Geometry: final body of the model. Coordinates: model frame, mm. A direction names the side the tool comes from. Give positions to 0.01 mm unless a question says otherwise; leave off trailing zeros. Write each loop counter-clockwise with the first axis right and the second up, starting at its lowest first coordinate (ties: lowest second). Pieces come first, ordered by that corner, then holes.
Q1. Cut plane C-C on y = 38. Return the cut outline in (x, z), plus the area to 3 significant figures.
Q2. Draft query along Z for faces 5 (the face through (99.254, 57.916, -4.251)), 6 (the face through (-38, 5, 16)), 7 (the face through (-39, 0, 0)), 8 (the face through (116, 41, -25)). Return one class per face: pulls with the +Z half, pulls with the -Z half, needs draft (parallel to the pull), parting line crosses it, or undercut.
Q3. Cut plane D-D on x = 120.5. Return the cut outline in (y, z).
Q4. Pin query (flat end, axial travel): pin 1 (11 mm diameter, centred on x = 91.5, y = 38.5, fed in from -Z); pin 2 (8 mm diameter, centred on y = 46, z = -12.5, fed in from -X); pin 3 (19 mm diameter, centred on x = 13.5, z = 35, fed in from -Y); pin 4 (18 mm diameter, centred on x = 89, z = 0, fed in from -Y). Return the tip coordinate at first contact, or that it passes through.
Q5. Line query: L1, parallel to Z at x = 0, y = 45; L2, parallel to Z at x = 89, y = 54; L3, parallel to Y at x = 21, z = -33.5. Output: solid intervals per line, ascending.
Q6. Cut plane A-A on x = 89. Return the cut outline in (y, z), plus the area to 3 significant figures.
Q7. Cut plane B-B on z = 0. Return the cut outline in (x, y), plus the area to 3 significant figures.
Q8. Reachability of faces 1 (the face through (-1, 10, -35)), 2 (the face through (38, 5, 16)), 3 (the face through (106, 47, 41)), 4 (the face through (60, 41, 0)) from +Z, -Z, +X, -X, +Y, -Y: full face, straight path, thin tool, end or side. Return the list, or none.
```python
from build123d import *

# Parameters (mm, degrees)
F0_R      = 54
F0_R_2    = 28.75
F1_DEPTH  = 64
F3_DEPTH  = 10
F4_R      = 11.1
F5_DEPTH  = 54
F6_DEPTH  = 20
F8_DEPTH  = 95.001
F9_W      = 114
F9_H      = 50
F10_DEPTH = 22


with BuildPart() as f1:
    # F0 (on Front) → F1 (new body)
    with BuildSketch(Plane.XZ):
        Circle(F0_R)
        Circle(F0_R_2, mode=Mode.SUBTRACT)
    extrude(amount=-F1_DEPTH)

    # F2 (on face) → F3 (cut)
    with BuildSketch(Plane.XZ):
        with BuildLine():
            ThreePointArc((23.88645, -16), (0, -28.75), (-23.88645, -16))
            Line((-23.88645, -16), (-51.575188, -16))
            ThreePointArc((-51.575188, -16), (0, -54), (51.575188, -16))
            Line((51.575188, -16), (23.88645, -16))
        make_face()
        with BuildLine():
            ThreePointArc((51.575188, 16), (0, 54), (-51.575188, 16))
            Line((-51.575188, 16), (-23.88645, 16))
            ThreePointArc((-23.88645, 16), (0, 28.75), (23.88645, 16))
            Line((23.88645, 16), (51.575188, 16))
        make_face()
    extrude(amount=-F3_DEPTH, mode=Mode.SUBTRACT)

    # F4 (on face) → F5 (join, through all)
    with BuildSketch(Plane.XZ.offset(-10)):
        with BuildLine():
            ThreePointArc((51.575188, -16), (45.124741, -29.660711), (35.142567, -41))
            Line((35.142567, -41), (174, -41))
            Line((174, -41), (174, 41))
            Line((174, 41), (35.142567, 41))
            ThreePointArc((35.142567, 41), (45.124741, 29.660711), (51.575188, 16))
            ThreePointArc((51.575188, 16), (54, 0), (51.575188, -16))
        make_face()
        with Locations((89, 0)):
            Circle(F4_R, mode=Mode.SUBTRACT)
        with Locations((139, 0)):
            Circle(F4_R, mode=Mode.SUBTRACT)
    extrude(amount=-F5_DEPTH)

    # F4 (on face) → F6 (cut)
    with BuildSketch(Plane.XZ.offset(-10)):
        with BuildLine():
            ThreePointArc((51.575188, -16), (45.124741, -29.660711), (35.142567, -41))
            Line((35.142567, -41), (174, -41))
            Line((174, -41), (174, 41))
            Line((174, 41), (35.142567, 41))
            ThreePointArc((35.142567, 41), (45.124741, 29.660711), (51.575188, 16))
            ThreePointArc((51.575188, 16), (54, 0), (51.575188, -16))
        make_face()
        with Locations((89, 0)):
            Circle(F4_R, mode=Mode.SUBTRACT)
        with Locations((139, 0)):
            Circle(F4_R, mode=Mode.SUBTRACT)
    extrude(amount=-F6_DEPTH, mode=Mode.SUBTRACT)

    # F7 (on face) → F8 (cut, through all)
    with BuildSketch(Plane.XY.offset(41)):
        Polygon((174, 42), (162, 30), (174, 30), align=None)
    extrude(amount=-F8_DEPTH, mode=Mode.SUBTRACT)

    # F9 (on face) → F10 (cut)
    with BuildSketch(Plane.XZ.offset(-30)):
        with Locations((117, 0)):
            Rectangle(F9_W, F9_H)
    extrude(amount=-F10_DEPTH, mode=Mode.SUBTRACT)


solid = f1.part
```
Data:
1. outline: (35.14, -41) - (170, -41) - (170, -25) - (60, -25) - (60, 25) - (170, 25) - (170, 41) - (35.14, 41) arc R54 ccw (long way) to start; hole circle Ø57.5 at (0, 0)
1. area: 11,000 mm2
2. face 5: undercut
2. face 6: pulls with the +Z half
2. face 7: needs draft
2. face 8: undercut
3. outline: (30, -41) - (64, -41) - (64, 41) - (30, 41) - (30, 25) - (52, 25) - (52, -25) - (30, -25) - close
4. pin 1: stops at z = -41
4. pin 2: stops at x = -53.33
4. pin 3: stops at y = 10
4. pin 4: passes through
5. L1: z = -54 to -28.75, 28.75 to 54
5. L2: z = -41 to -11.1, 11.1 to 41
5. L3: y = 10 to 64
6. outline: (30, -41) - (64, -41) - (64, -11.1) - (52, -11.1) - (52, -25) - (30, -25) - close; (30, 25) - (52, 25) - (52, 11.1) - (64, 11.1) - (64, 41) - (30, 41) - close
6. area: 1,420 mm2
7. outline: (-54, 0) - (-28.75, 0) - (-28.75, 64) - (-54, 64) - close; (28.75, 0) - (54, 0) - (54, 30) - (60, 30) - (60, 52) - (77.9, 52) - (77.9, 64) - (28.75, 64) - close; (100.1, 52) - (127.9, 52) - (127.9, 64) - (100.1, 64) - close; (150.1, 52) - (174, 52) - (174, 64) - (150.1, 64) - close
7. area: 4,270 mm2
8. face 1: -Z, +X, -X, -Y
8. face 2: +Z, +X, -X, -Y
8. face 3: +Z, +X, +Y, -Y
8. face 4: +X, -Y
